Could you check a few things on this model? Use its own coordinates, in mm. Face numbers are marked on the shaded views. Coordinates: 2 decimals unless noted, no trailing zeros. Write each loop counter-clockwise with the first axis right and the second up, starting at its lowest first coordinate (ties: lowest second). Pieces come first, ordered by that corner, then holes. Notation, with made-up numbers: M 58.25,69 L 79.25,69 A24 ccw 79.25,84 Z; hole C 40.25,-9 d11. An arc over 180 degrees is marked long. Answer as CSV lines item,"result". Start each with the question number.
Item 1: Suppose I cut it at B-B, the plane z = 70. Write out the boundary of the cut face in (x, y).
Item 2: Suppose I cut it at D-D, the plane y = 21. Write out the boundary of the cut face in (x, z).
Item 3: Suppose I cut it at C-C, the plane x = 64. Write out the boundary of the cut face in (y, z), and give its area (3 significant figures).
Item 4: If I drill on line 1 along Y through (x, z) = (0, 1.1); line 2 along Y through (x, z) = (-92.5, 3.75); line 3 along X through (y, z) = (-5, 23), over which ranges is the centre line in solid material (lowest first)? Write a range as [from, to].
Item 5: Suppose I cut it at A-A, the plane z = 59. Write out the boundary of the cut face in (x, y), and give its area (3 significant figures).
Item 6: We'd pull the mould along Y, two halves only. Please class the marked faces 1, 2, 3 and 4: +Y half, -Y half, draft (parallel to the pull), parting line (faces both ways), or undercut.
Item 7: I'm going to push flat-ended pins straight in: P1, Ø1.2, axis at x = -91.5, y = -27.5, coming from the +Z side; P2, Ø2.5, axis at x = 102.5, y = 57.5, coming from the +Z side; P3, Ø8, axis at x = -36.5, y = 33, coming from the +Z side; P4, Ø6, axis at x = -76.5, y = -12.5, coming from the -Z side. Where does each tip first touch, or does it pass through?
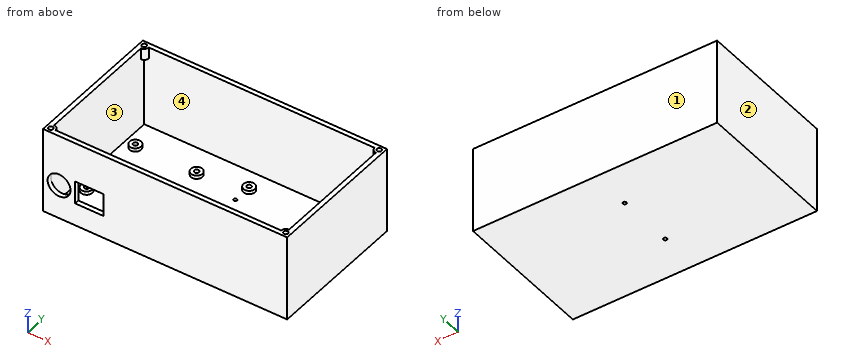
```python
from build123d import *

# Parameters (mm, degrees)
SKETCH1_W                           = 205
SKETCH1_H                           = 115
BOSS_EXTRUDE1_DEPTH                 = 3
SKETCH2_R                           = 5
SKETCH2_R_2                         = 2
BOSS_EXTRUDE2_DEPTH                 = 3
SKETCH3_R                           = 5
SKETCH3_R_2                         = 2
BOSS_EXTRUDE3_DEPTH                 = 3
SKETCH5_W                           = 213
SKETCH5_H                           = 123
SKETCH5_W_2                         = 205
SKETCH5_H_2                         = 115
BOSS_EXTRUDE4_DEPTH                 = 75
F_3_0MM_CLEARANCE_DOWEL_HOLE1_D     = 3
F_3_0MM_CLEARANCE_DOWEL_HOLE1_DEPTH = 30
F_3_0MM_CLEARANCE_DOWEL_HOLE1_TIP   = 0.901290929
SKETCH10_W                          = 25
SKETCH10_H                          = 20
CUT_EXTRUDE1_DEPTH                  = 4
SKETCH11_R                          = 10
CUT_EXTRUDE2_DEPTH                  = 4
SKETCH12_R                          = 4
SKETCH12_R_2                        = 2
BOSS_EXTRUDE5_DEPTH                 = 10
SKETCH13_R                          = 2
CUT_EXTRUDE3_DEPTH                  = 10


with BuildPart() as part:
    # Sketch1 → Boss-Extrude1 (new body)
    with BuildSketch(Plane.XY):
        Rectangle(SKETCH1_W, SKETCH1_H)
    extrude(amount=BOSS_EXTRUDE1_DEPTH)

    # Sketch2 → Boss-Extrude2 (add)
    with BuildSketch(Plane.XY.offset(3)):
        with Locations((-92.5, 32.5)):
            Circle(SKETCH2_R)
        with Locations((-92.5, 32.5)):
            Circle(SKETCH2_R_2, mode=Mode.SUBTRACT)
        with Locations((-92.5, -27.5)):
            Circle(SKETCH2_R)
        with Locations((-92.5, -27.5)):
            Circle(SKETCH2_R_2, mode=Mode.SUBTRACT)
        with Locations((-39, 32.5)):
            Circle(SKETCH2_R)
        with Locations((-39, 32.5)):
            Circle(SKETCH2_R_2, mode=Mode.SUBTRACT)
        with Locations((-39, -27.5)):
            Circle(SKETCH2_R)
        with Locations((-39, -27.5)):
            Circle(SKETCH2_R_2, mode=Mode.SUBTRACT)
    extrude(amount=BOSS_EXTRUDE2_DEPTH)

    # Sketch3 → Boss-Extrude3 (add)
    with BuildSketch(Plane.XY.offset(3)):
        with Locations((1.5, 40)):
            Circle(SKETCH3_R)
        with Locations((1.5, 40)):
            Circle(SKETCH3_R_2, mode=Mode.SUBTRACT)
        with Locations((82.5, -36)):
            Circle(SKETCH3_R)
        with Locations((82.5, -36)):
            Circle(SKETCH3_R_2, mode=Mode.SUBTRACT)
        with Locations((82.5, 40)):
            Circle(SKETCH3_R)
        with Locations((82.5, 40)):
            Circle(SKETCH3_R_2, mode=Mode.SUBTRACT)
        with Locations((1.5, -36)):
            Circle(SKETCH3_R)
        with Locations((1.5, -36)):
            Circle(SKETCH3_R_2, mode=Mode.SUBTRACT)
    extrude(amount=BOSS_EXTRUDE3_DEPTH)

    # Sketch5 → Boss-Extrude4 (add)
    with BuildSketch(Plane(origin=(0, 0, 0), x_dir=(-1, 0, 0), z_dir=(0, 0, -1))):
        Rectangle(SKETCH5_W, SKETCH5_H)
        Rectangle(SKETCH5_W_2, SKETCH5_H_2, mode=Mode.SUBTRACT)
    extrude(amount=-BOSS_EXTRUDE4_DEPTH)

    # Ø3.0mm Clearance Dowel Hole1
    with Locations(Plane.XY.offset(3)):
        with Locations((0, 25), (0, -25)):
            Hole(F_3_0MM_CLEARANCE_DOWEL_HOLE1_D / 2, depth=F_3_0MM_CLEARANCE_DOWEL_HOLE1_DEPTH)
            with Locations((0, 0, -(F_3_0MM_CLEARANCE_DOWEL_HOLE1_DEPTH + F_3_0MM_CLEARANCE_DOWEL_HOLE1_TIP / 2))):  # 118° drill point
                Cone(0, F_3_0MM_CLEARANCE_DOWEL_HOLE1_D / 2, F_3_0MM_CLEARANCE_DOWEL_HOLE1_TIP, mode=Mode.SUBTRACT)

    # Sketch10 → Cut-Extrude1 (cut)
    with BuildSketch(Plane.XZ.offset(61.5)):
        with Locations((-66, 30)):
            Rectangle(SKETCH10_W, SKETCH10_H)
    extrude(amount=-CUT_EXTRUDE1_DEPTH, mode=Mode.SUBTRACT)

    # Sketch11 → Cut-Extrude2 (cut)
    with BuildSketch(Plane.XZ.offset(61.5)):
        with Locations((-92.5, 30)):
            Circle(SKETCH11_R)
    extrude(amount=-CUT_EXTRUDE2_DEPTH, mode=Mode.SUBTRACT)

    # Sketch12 → Boss-Extrude5 (add)
    with BuildSketch(Plane.XY.offset(75)):
        with Locations((102.5, -57.5)):
            Circle(SKETCH12_R)
        with Locations((102.5, -57.5)):
            Circle(SKETCH12_R_2, mode=Mode.SUBTRACT)
        with Locations((102.5, 57.5)):
            Circle(SKETCH12_R)
        with Locations((-102.5, 57.5)):
            Circle(SKETCH12_R)
        with Locations((-102.5, -57.5)):
            Circle(SKETCH12_R)
    extrude(amount=-BOSS_EXTRUDE5_DEPTH)

    # Sketch13 → Cut-Extrude3 (cut)
    with BuildSketch(Plane.XY.offset(75)):
        with Locations((102.5, -57.5)):
            Circle(SKETCH13_R)
        with Locations((102.5, 57.5)):
            Circle(SKETCH13_R)
        with Locations((-102.5, 57.5)):
            Circle(SKETCH13_R)
        with Locations((-102.5, -57.5)):
            Circle(SKETCH13_R)
    extrude(amount=-CUT_EXTRUDE3_DEPTH, mode=Mode.SUBTRACT)


solid = part.part
```
Ans:
1,outline,"M -106.5,-61.5 L 106.5,-61.5 L 106.5,61.5 L -106.5,61.5 Z; hole C -102.5,-57.5 d4; hole C -102.5,57.5 d4; hole M -102.5,-53.5 A4 cw -98.5,-57.5 L 98.5,-57.5 A4 cw 102.5,-53.5 L 102.5,53.5 A4 cw 98.5,57.5 L -98.5,57.5 A4 cw -102.5,53.5 Z; hole C 102.5,-57.5 d4; hole C 102.5,57.5 d4"
2,outline,"M -106.5,0 L 106.5,0 L 106.5,75 L 102.5,75 L 102.5,3 L -102.5,3 L -102.5,75 L -106.5,75 Z"
3,outline,"M -61.5,0 L 61.5,0 L 61.5,75 L 57.5,75 L 57.5,3 L -57.5,3 L -57.5,75 L -61.5,75 Z"
3,area,"945 mm^2"
4,line 1,"y = [-61.5, -26.5], [-23.5, 23.5], [26.5, 61.5]"
4,line 2,"y = [-61.5, -57.5], [-32.5, -29.5], [-25.5, -22.5], [27.5, 30.5], [34.5, 37.5], [57.5, 61.5]"
4,line 3,"x = [-106.5, -102.5], [102.5, 106.5]"
5,outline,"M -106.5,-61.5 L 106.5,-61.5 L 106.5,61.5 L -106.5,61.5 Z; hole M -102.5,-57.5 L 102.5,-57.5 L 102.5,57.5 L -102.5,57.5 Z"
5,area,"2,620 mm^2"
6,face 1,"+Y half"
6,face 2,"draft"
6,face 3,"undercut"
6,face 4,"undercut"
7,P1,"stops at z = 3"
7,P2,"stops at z = 65"
7,P3,"stops at z = 6"
7,P4,"stops at z = 0"
